Could you check a few things on this model? Use its own coordinates, in mm. A direction names the side the tool comes from. Give positions to 0.01 mm unless a question says otherwise; leave off trailing zeros. Write each loop counter-clockwise with the first axis right and the second up, starting at its lowest first coordinate (ties: lowest second). Pieces come first, ordered by that corner, then holes. Notation, with made-up numbers: (-2, 15) - (31, 15) arc R14 ccw to (31, 42) - close; hole circle Ø8 at (-30.75, 79.25). An arc over 180 degrees is marked (long way). Answer in a Markdown table with one row per item.
from build123d import *

# Parameters (mm, degrees)
CROQUIS1_W              = 140.396098848
CROQUIS1_H              = 71.000312846
SALIENTE_EXTRUIR1_DEPTH = 10
VACIADO1_T              = -0.5
EXTRUIR_L_MINA1_DEPTH   = 0.8


with BuildPart() as part:
    # Croquis1 → Saliente-Extruir1 (new body)
    with BuildSketch(Plane(origin=(0, 0, 0), x_dir=(1, 0, 0), z_dir=(0, 1, 0))):
        with Locations((-70.198049424, -32.892800302)):
            Rectangle(CROQUIS1_W, CROQUIS1_H)
    extrude(amount=SALIENTE_EXTRUIR1_DEPTH)

    # Vaciado1
    vaciado1_openings = [part.faces().sort_by_distance(p)[0] for p in [
        (-70.198049424, 10, 32.892800302),
    ]]
    offset(amount=VACIADO1_T, openings=vaciado1_openings, kind=Kind.INTERSECTION)

    # Croquis2 → Extruir-Lámina1 (add)
    with BuildSketch(Plane(origin=(0, 0, 0), x_dir=(1, 0, 0), z_dir=(0, 1, 0))):
        with BuildLine():
            ThreePointArc((-0.5, -21.806712241), (10.724107373, -32.530819614), (0, -43.754926987))
            Line((0, -43.754926987), (-0.227749871, -33.757520824))
            ThreePointArc((-0.227749871, -33.757520824), (0.72670121, -32.758569485), (-0.272250129, -31.804118404))
            Line((-0.272250129, -31.804118404), (-0.5, -21.806712241))
        make_face()
    extrude(amount=EXTRUIR_L_MINA1_DEPTH)


solid = part.part
1) Imagine slicing it at C-C (z = 6). List the corners of the cut face in (x, y) for me.
Check values:
| item | result |
|---|---|
| outline | (-140.4, 0) - (0, 0) - (0, 10) - (-0.5, 10) - (-0.5, 0.5) - (-139.9, 0.5) - (-139.9, 10) - (-140.4, 10) - close |
2) Imagine slicing it at D-D (z = 35.5). List the corners of the cut face in (x, y) for me, then the cut area to 3 significant figures.
Check values:
| item | result |
|---|---|
| outline | (-140.4, 0) - (10.38, 0) - (10.38, 0.8) - (0, 0.8) - (0, 10) - (-0.5, 10) - (-0.5, 0.5) - (-139.9, 0.5) - (-139.9, 10) - (-140.4, 10) - close |
| area | 88.0 mm2 |
3) If I drill on line 1 (X direction, y = 7.5, z = 13.5); line 2 (Z direction, x = -122, y = 9); line 3 (Y direction, x = -97, z = 40), over which ranges is the centre line in solid material (lowest first)?
Check values:
| item | result |
|---|---|
| line 1 | x = -140.4 to -139.9, -0.5 to 0 |
| line 2 | z = -2.61 to -2.11, 67.89 to 68.39 |
| line 3 | y = 0 to 0.5 |
4) On a 3-axis mill with a long thin cutter (end or side, diameter ignored), from which of +Z, -Z, +X, -X, +Y, -Y can I reach the whole of each face in a straight line? I mean faces 1 (the face through (-71, 5, -2.107)), 2 (the face through (10.724, 0.394, 32.543)). Say none if no direction works.
Check values:
| item | result |
|---|---|
| face 1 | +Y |
| face 2 | +X, +Y, -Y |
5) Imagine slicing it at B-B (x = -86). List the corners of the cut face in (y, z) for me.
Check values:
| item | result |
|---|---|
| outline | (0, -2.61) - (10, -2.61) - (10, -2.11) - (0.5, -2.11) - (0.5, 67.89) - (10, 67.89) - (10, 68.39) - (0, 68.39) - close |
6) Imagine slicing it at A-A (y = 7.75). List the corners of the cut face in (x, z) for me.
Check values:
| item | result |
|---|---|
| outline | (-140.4, -2.61) - (0, -2.61) - (0, 68.39) - (-140.4, 68.39) - close; hole (-139.9, -2.11) - (-0.5, -2.11) - (-0.5, 67.89) - (-139.9, 67.89) - close |
7) Will these pins go through, and if not, where does the flat tip stop? P1, Ø8, axis at x = -18, z = 5.5, coming from the +Y side; P2, Ø3, axis at y = 7.5, z = 53, coming from the +X side; P3, Ø12, axis at x = 5.5, z = 29, coming from the +Y side.
Check values:
| item | result |
|---|---|
| P1 | stops at y = 0.5 |
| P2 | stops at x = 0 |
| P3 | stops at y = 10 |
8) We'd pull the mould along Z, two halves only. Please class faces 3 (the face through (4, 0.8, 33)), 4 (the face through (-0.5, 5, 33)), 5 (the face through (-71, 5, 67.893)), 6 (the face through (-71, 5, 68.393)): +Z half, -Z half, draft (parallel to the pull), parting line (faces both ways), or undercut.
Check values:
| item | result |
|---|---|
| face 3 | draft |
| face 4 | undercut |
| face 5 | undercut |
| face 6 | +Z half |
